Part model, mm, in its own coordinate system. Face numbers are marked on the shaded views. A direction names the side the tool comes from. Round coordinates to 2 decimals unless told otherwise and drop trailing zeros. Loops run counter-clockwise (first coordinate to the right, second up) from the corner with the lowest first, then second, coordinate; pieces in that order, holes last. Notation, with made-up numbers: (44.25, 82) - (59.25, 82) arc R14 ccw to (59.25, 108) - close; hole circle Ø1 at (77, 43). An arc over 180 degrees is marked (long way). Put each result on its own line as item: value.
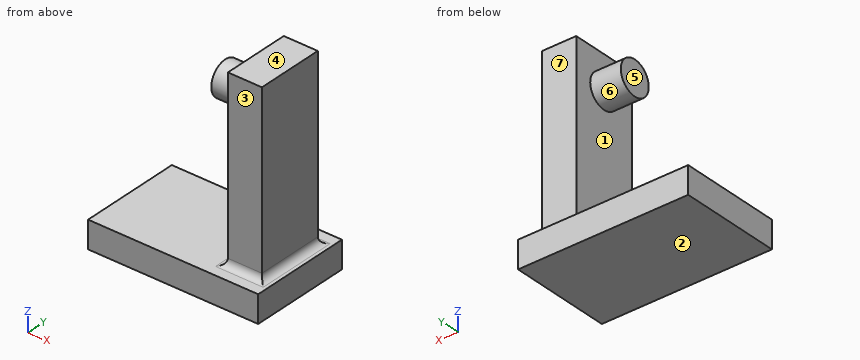
from build123d import *

# Parameters (mm, degrees)
CYLINDER024_R     = 2.5
CYLINDER024_DEPTH = 5
BOX023_W          = 5
BOX023_H          = 10
BOX023_DEPTH      = 30
BOX024_W          = 25
BOX024_H          = 15
BOX024_DEPTH      = 4
FILLET_R          = 1


with BuildPart() as obj1:
    # Cylinder024 → Cylinder024 (new body)
    with BuildSketch(Plane(origin=(92, 2.5, 30), x_dir=(0, 0, -1), z_dir=(1, 0, 0))):
        Circle(CYLINDER024_R)
    extrude(amount=CYLINDER024_DEPTH)


with BuildPart() as obj2:
    # Box023 → Box023 (new body)
    with BuildSketch(Plane(origin=(96.5, -2.5, 5), x_dir=(1, 0, 0), z_dir=(0, 0, 1))):
        with Locations((2.5, 5)):
            Rectangle(BOX023_W, BOX023_H)
    extrude(amount=BOX023_DEPTH)

    # Fusion016: union obj1
    add(obj1.part)


with BuildPart() as obj3:
    # Box024 → Box024 (new body)
    with BuildSketch(Plane(origin=(78, -5, 5), x_dir=(1, 0, 0), z_dir=(0, 0, 1))):
        with Locations((12.5, 7.5)):
            Rectangle(BOX024_W, BOX024_H)
    extrude(amount=BOX024_DEPTH)

    # Fusion017: union obj2
    add(obj2.part)


with BuildPart() as obj3_1:
    # Fusion017 placement: moved
    add(obj3.part.moved(Location((-4, 0, 0))))

    # Fillet
    fillet_edges = [obj3_1.edges().sort_by_distance(p)[0] for p in [
        (95, -2.5, 9),
        (97.5, 2.5, 9),
        (95, 7.5, 9),
        (92.5, 2.5, 9),
    ]]
    fillet(fillet_edges, radius=FILLET_R)


solid = obj3_1.part
1. Band-saw the part on D-D (y = 6.5). List the corners of the cut face in (x, z), plus the area to 3 significant figures.
A:
outline: (74, 5) - (99, 5) - (99, 9) - (98.5, 9) arc R1 cw to (97.5, 10) - (97.5, 35) - (92.5, 35) - (92.5, 10) arc R1 cw to (91.5, 9) - (74, 9) - close
area: 230 mm²
2. Pin check, flat tips, straight feed: P1, Ø2.5, axis at x = 95.5, z = 28, coming from the +Y side; P2, Ø5, axis at y = 4, z = 19.5, coming from the -X side; P3, Ø12, axis at x = 86, z = 30.5, coming from the -Y side. Stop position of each tip, or through.
A:
P1: stops at y = 7.5
P2: stops at x = 92.5
P3: stops at y = 0
3. Band-saw the part on C-C (x = 93.75). List the corners of the cut face in (y, z), plus the area to 3 significant figures.
A:
outline: (-5, 5) - (10, 5) - (10, 9) - (8.5, 9) arc R1 cw to (7.5, 10) - (7.5, 35) - (-2.5, 35) - (-2.5, 10) arc R1 cw to (-3.5, 9) - (-5, 9) - close
area: 320 mm²
4. Two-plate mould, pull along Z, no slides. Class the marked faces 1, 2, 3 and 4: pulls with the +Z half, pulls with the -Z half, needs draft (parallel to the pull), parting line crosses it, or undercut.
A:
face 1: undercut
face 2: pulls with the -Z half
face 3: needs draft
face 4: pulls with the +Z half
5. Band-saw the part on B-B (y = 2.5). List the corners of the cut face in (x, z), plus the area to 3 significant figures.
A:
outline: (74, 5) - (99, 5) - (99, 9) - (98.5, 9) arc R1 cw to (97.5, 10) - (97.5, 35) - (92.5, 35) - (92.5, 32.5) - (88, 32.5) - (88, 27.5) - (92.5, 27.5) - (92.5, 10) arc R1 cw to (91.5, 9) - (74, 9) - close
area: 253 mm²
6. Tool access for the marked faces 5, 6 and 7: list every direction of +Z, -Z, +X, -X, +Y, -Y with a clear straight run to the whole face (end or side of a thin tool).
A:
face 5: +Z, -X, +Y, -Y
face 6: -X
face 7: +Z, +X, -X, +Y
7. Probe line 1 along Y through (x, z) = (94.5, 21.25); line 2 along X through (y, z) = (1.75, 14.25); line 3 along Z through (x, y) = (81.75, 4.5). List the from-to ranges inside material, lowest first. Write a range as [from, to].
A:
line 1: y = [-2.5, 7.5]
line 2: x = [92.5, 97.5]
line 3: z = [5, 9]
8. Band-saw the part on A-A (z = 30). List the corners of the cut face in (x, y), plus the area to 3 significant figures.
A:
outline: (88, 0) - (92.5, 0) - (92.5, -2.5) - (97.5, -2.5) - (97.5, 7.5) - (92.5, 7.5) - (92.5, 5) - (88, 5) - close
area: 72.5 mm²
